Read the model definition and answer for the solid it produces. Units are mm, in the model's axes. A direction names the side the tool comes from. Coordinates: 2 decimals unless noted, no trailing zeros. Write each loop counter-clockwise with the first axis right and the second up, starting at its lowest first coordinate (ties: lowest second). Pieces come first, ordered by that corner, then holes.
1) The part is cut by section A-A (z = 2.75). Determine the outline of the cut face in (x, y).
2) Find the intervals of material crossed by line 1 (Z direction, x = -10, y = -0.8); line 2 (X direction, y = -0.55, z = 0); line 3 (X direction, y = 0.5, z = -1), in increasing order.
3) Each of these flat-tipped pins is pushed along its axis until it touches: pin 1 Ø0.5 at (x, z) = (-6.5, -0.5) entering from +Y; pin 2 Ø1.1 at (x, z) = (-5, 0.5) entering from +Y; pin 3 Ø1 at (y, z) = (6, 0) entering from -X; pin 4 Ø3 at (x, y) = (0, 2.65) entering from +Z. Where does it stop, or does it pass through?
4) The part is cut by section B-B (y = -0.25). Determine the outline of the cut face in (x, z).
5) Determine the mould class of faces 1 (the face through (-12, 0, 0)), 2 (the face through (-10.74, 6.53, -0.07)), 3 (the face through (-10.35, -0.35, -1.56)), 4 (the face through (-11.6, 0.8, -0.9)) for opening direction X: +X half, -X half, draft (parallel to the pull), parting line (faces both ways), or undercut.
6) The part is cut by section C-C (x = -6.25). Determine the outline of the cut face in (y, z), then the cut area to 3 significant figures.
7) Which of the six approach directions +Z, -Z, +X, -X, +Y, -Y give full straight-line access (tool end or side, diameter ignored) to faces 5 (the face through (-6, 0.8, 4)), 6 (the face through (-6, 0.8, -3)), 7 (the face through (-6.79, 4.48, 0.07)), 8 (the face through (-4, 1, -5))?
8) The part is cut by section D-D (z = -0.5). Determine the outline of the cut face in (x, y), then the cut area to 3 significant figures.
from build123d import *

# Parameters (mm, degrees)
BOSS_EXTRUDE1_DEPTH      = 5
CUT_EXTRUDE5_REACH       = 11.607
SKETCH4_R                = 1.6
CUT_EXTRUDE6_REACH       = 11.612
SKETCH5_R                = 1.6
CUT_EXTRUDE12_DEPTH      = 1
CUT_EXTRUDE12_DEPTH_BACK = 12


with BuildPart() as part:
    # Sketch1 → Boss-Extrude1 (new body, symmetric)
    with BuildSketch(Plane.XY):
        with BuildLine():
            Line((4, 6.083853012), (-11.403967093, 8.111823753))
            Line((-11.403967093, 8.111823753), (-11.795545669, 5.137489168))
            Line((-11.795545669, 5.137489168), (-1.636306817, 3.8))
            ThreePointArc((-1.636306817, 3.8), (2, 2.65), (-1.636306817, 1.5))
            Line((-1.636306817, 1.5), (-12, 1.5))
            Line((-12, 1.5), (-12, -1.5))
            Line((-12, -1.5), (4, -1.5))
            Line((4, -1.5), (4, 6.083853012))
        make_face()
    extrude(amount=BOSS_EXTRUDE1_DEPTH, both=True)

    # Sketch4 → Cut-Extrude5 (cut, up to next)
    with BuildSketch(Plane(origin=(0.855456861, 6.49783997, 0), x_dir=(0.991444861, -0.130526192, 0), z_dir=(0.130526192, 0.991444861, 0)), mode=Mode.PRIVATE) as cut_extrude5_sk1:
        with Locations((-9.9, 0)):
            Circle(SKETCH4_R)
    cut_extrude5_tool1 = extrude(cut_extrude5_sk1.sketch, amount=-CUT_EXTRUDE5_REACH, mode=Mode.PRIVATE) & part.part
    add(cut_extrude5_tool1.solids().sort_by_distance((-8.959847, 7.790049, 0))[0], mode=Mode.SUBTRACT)

    # Sketch5 → Cut-Extrude6 (cut, up to next)
    with BuildSketch(Plane.XZ.offset(1.5), mode=Mode.PRIVATE) as cut_extrude6_sk1:
        with Locations((-10, 0)):
            Circle(SKETCH5_R)
    cut_extrude6_tool1 = extrude(cut_extrude6_sk1.sketch, amount=-CUT_EXTRUDE6_REACH, mode=Mode.PRIVATE) & part.part
    add(cut_extrude6_tool1.solids().sort_by_distance((-10, -1.5, 0))[0], mode=Mode.SUBTRACT)

    # Sketch6 → Cut-Extrude12 (cut, two sides)
    with BuildSketch(Plane.ZY.offset(12)) as cut_extrude12_sk:
        Polygon((-2.5, 1.5), (-4, 1.5), (-3.745220836, 0.8), (-2.754779164, 0.8), align=None)
        Polygon((0, 1.5), (-1.5, 1.5), (-1.245220836, 0.8), (-0.254779164, 0.8), align=None)
        Polygon((3.754779164, 0.8), (5, 0.8), (5, 1.5), (3.5, 1.5), align=None)
        Polygon((2.5, 1.5), (1, 1.5), (1.254779164, 0.8), (2.245220836, 0.8), align=None)
    extrude(amount=CUT_EXTRUDE12_DEPTH, mode=Mode.SUBTRACT)
    extrude(cut_extrude12_sk.sketch, amount=-CUT_EXTRUDE12_DEPTH_BACK, mode=Mode.SUBTRACT)


solid = part.part
Reported:
1. outline: (-12, -1.5) - (4, -1.5) - (4, 6.08) - (-11.4, 8.11) - (-11.8, 5.14) - (-1.64, 3.8) arc R2 cw (long way) to (-1.64, 1.5) - (-12, 1.5) - close
2. line 1: z = -5 to -1.6, 1.6 to 5
2. line 2: x = -12 to -11.6, -8.4 to 4
2. line 3: x = -12 to -11.25, -8.75 to 4
3. pin 1: stops at y = 7.5
3. pin 2: stops at y = 7.34
3. pin 3: stops at x = -11.75
3. pin 4: passes through
4. outline: (-12, -5) - (4, -5) - (4, 5) - (-12, 5) - close; hole circle Ø3.2 at (-10, 0)
5. face 1: -X half
5. face 2: undercut
5. face 3: undercut
5. face 4: draft
6. outline: (-1.5, -5) - (1.5, -5) - (1.5, -4) - (0.8, -3.75) - (0.8, -2.75) - (1.5, -2.5) - (1.5, -1.5) - (0.8, -1.25) - (0.8, -0.25) - (1.5, 0) - (1.5, 1) - (0.8, 1.25) - (0.8, 2.25) - (1.5, 2.5) - (1.5, 3.5) - (0.8, 3.75) - (0.8, 5) - (-1.5, 5) - close; (4.41, -5) - (7.43, -5) - (7.43, 5) - (4.41, 5) - close
6. area: 56.7 mm2
7. face 5: +Z, -X
7. face 6: -X
7. face 7: +Z, -Z, -X
7. face 8: -Z, +X, -X, +Y, -Y
8. outline: (-12, -1.5) - (-11.52, -1.5) - (-11.52, 0.8) - (-12, 0.8) - close; (-11.8, 5.14) - (-10.86, 5.01) - (-10.47, 7.99) - (-11.4, 8.11) - close; (-8.48, -1.5) - (4, -1.5) - (4, 6.08) - (-7.45, 7.59) - (-7.84, 4.62) - (-1.64, 3.8) arc R2 cw (long way) to (-0.76, 0.8) - (-8.48, 0.8) - close
8. area: 70.5 mm2
